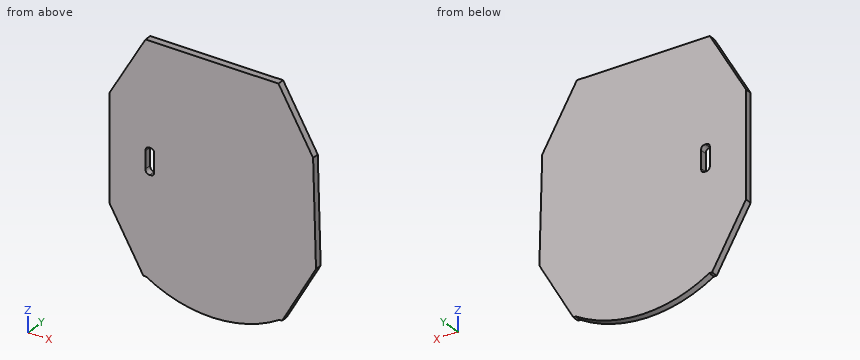
```python
from build123d import *

# Parameters (mm, degrees)
SKETCH2_W           = 2
SKETCH2_H           = 6
BOSS_EXTRUDE1_DEPTH = 1.6
FILLET1_SIZE        = 1


with BuildPart() as part:
    # Sketch2 → Boss-Extrude1 (new body)
    with BuildSketch(Plane(origin=(0, 0, 0), x_dir=(1, 0, 0), z_dir=(0, 1, 0))):
        with BuildLine():
            Line((-123.876706844, -10.393367026), (-123.876706844, -34.615283413))
            Line((-123.876706844, -34.615283413), (-115.532924627, -49.06713814))
            Line((-115.532924627, -49.06713814), (-84.860830246, -49.06713814))
            Line((-84.860830246, -49.06713814), (-76.867006735, -35.221429673))
            Line((-76.867006735, -35.221429673), (-76.19895922, -10.944023897))
            Line((-76.19895922, -10.944023897), (-84.03338266, 2.952288601))
            Line((-84.03338266, 2.952288601), (-84.615952241, 2.956571663))
            ThreePointArc((-84.615952241, 2.956571663), (-99.977425615, 7.344868085), (-115.401760623, 3.182909496))
            Line((-115.401760623, 3.182909496), (-116.035748857, 3.187570589))
            Line((-116.035748857, 3.187570589), (-123.876706844, -10.393367026))
        make_face()
        with Locations((-114.526706844, -22.504325219)):
            Rectangle(SKETCH2_W, SKETCH2_H, mode=Mode.SUBTRACT)
    extrude(amount=BOSS_EXTRUDE1_DEPTH)

    # Fillet1
    # a fillet whose section is not a circle: 1 mm, written as the material it adds along each edge
    with BuildSketch(Plane(origin=(-113.526706844, 0, 25.504325219), x_dir=(0, 0, -1), z_dir=(0, 1, 0)), Plane(origin=(-115.526706844, 0, 25.504325219), x_dir=(1, 0, 0), z_dir=(0, 1, 0)), Plane(origin=(-115.526706844, 0, 19.504325219), x_dir=(0, 0, 1), z_dir=(0, 1, 0))) as fillet1_piece_1:
        with BuildLine():
            add(Edge.make_bspline([(FILLET1_SIZE, 0), (FILLET1_SIZE * 0.831801948466, 0), (FILLET1_SIZE * 0.663603896932, 0), (FILLET1_SIZE * 0.292893218813, FILLET1_SIZE * 0.0716919198361), (FILLET1_SIZE * 0.0716919198361, FILLET1_SIZE * 0.292893218813), (0, FILLET1_SIZE * 0.663603896932), (0, FILLET1_SIZE * 0.831801948466), (0, FILLET1_SIZE)], knots=[0, 0, 0, 0, 0, 0, 0.5, 0.5, 1, 1, 1, 1, 1, 1], degree=5))
            Line((0, FILLET1_SIZE), (-FILLET1_SIZE * 0.02, FILLET1_SIZE))
            Line((-FILLET1_SIZE * 0.02, FILLET1_SIZE), (-FILLET1_SIZE * 0.02, -FILLET1_SIZE * 0.02))
            Line((-FILLET1_SIZE * 0.02, -FILLET1_SIZE * 0.02), (FILLET1_SIZE, -FILLET1_SIZE * 0.02))
            Line((FILLET1_SIZE, -FILLET1_SIZE * 0.02), (FILLET1_SIZE, 0))
        make_face()
    extrude(amount=1.6)
    with BuildSketch(Plane(origin=(-113.526706844, 0, 19.504325219), x_dir=(0, 0, 1), z_dir=(0, 1, 0))) as fillet1_piece_2:
        with BuildLine():
            add(Edge.make_bspline([(FILLET1_SIZE, 0), (FILLET1_SIZE * 0.831801948466, 0), (FILLET1_SIZE * 0.663603896932, 0), (FILLET1_SIZE * 0.292893218813, -FILLET1_SIZE * 0.0716919198361), (FILLET1_SIZE * 0.0716919198361, -FILLET1_SIZE * 0.292893218813), (0, -FILLET1_SIZE * 0.663603896932), (0, -FILLET1_SIZE * 0.831801948466), (0, -FILLET1_SIZE)], knots=[0, 0, 0, 0, 0, 0, 0.5, 0.5, 1, 1, 1, 1, 1, 1], degree=5))
            Line((0, -FILLET1_SIZE), (-FILLET1_SIZE * 0.02, -FILLET1_SIZE))
            Line((-FILLET1_SIZE * 0.02, -FILLET1_SIZE), (-FILLET1_SIZE * 0.02, FILLET1_SIZE * 0.02))
            Line((-FILLET1_SIZE * 0.02, FILLET1_SIZE * 0.02), (FILLET1_SIZE, FILLET1_SIZE * 0.02))
            Line((FILLET1_SIZE, FILLET1_SIZE * 0.02), (FILLET1_SIZE, 0))
        make_face()
    extrude(amount=1.6)


solid = part.part
```
Could you check a few things on this model? Use its own coordinates, in mm. Round coordinates to 2 decimals unless told otherwise and drop trailing zeros. Order: outer loops, then holes, each group sorted by start corner. A loop starts at its lowest first (then second) coordinate and runs counter-clockwise, first axis right, second up. Notation, with made-up numbers: M -15.5,16 L 8.5,16 A17 ccw 8.5,29 Z; hole C -21,35.25 d2. An arc over 180 degrees is marked long. One line per question, with ' | ' between items. Start each with the question number.
(1) Please list where these lines run through material, in increasing order: line 1 along X through (y, z) = (0.6, 11); line 2 along X through (y, z) = (0.8, 24); line 3 along Z through (x, y) = (-99, 1.2).
(2) Suppose I cut it at B-B on z = 1. List the corners of the cut face in (x, y) for me.
(3) Suppose I cut it at A-A on x = -117.5. List the corners of the cut face in (y, z) for me, then the cut area to 3 significant figures.
(4) For P1, Ø0.8, axis at y = 0.5, z = 22, coming from the +X side; P2, Ø8, axis at x = -98.5, z = 13, coming from the -Y side, each with a flat end and sliding along its axis, tell me the tip position at first contact or that it passes through.
Geometry results:
1) line 1: -123.88 to -76.2 | line 2: -123.88 to -115.53, -113.53 to -76.56 | line 3: -7.32 to 49.07
2) outline: M -118.45,0 L -81.81,0 L -81.81,1.6 L -118.45,1.6 Z
3) outline: M 0,-0.65 L 1.6,-0.65 L 1.6,45.66 L 0,45.66 Z | area: 74.1 mm²
4) P1: x = -76.49 | P2: y = 0
